Design review of the part built by this model. Coordinates are the model's own, in mm. Face numbers are marked on the shaded views. A direction names the side the tool comes from. Give positions to 0.01 mm unless a question says otherwise; leave off trailing zeros. Write each loop counter-clockwise with the first axis right and the second up, starting at its lowest first coordinate (ties: lowest second). Pieces come first, ordered by that corner, then holes.
```python
from build123d import *
from OCP.BRepFilletAPI import BRepFilletAPI_MakeChamfer

# Parameters (mm, degrees)
SKETCH1_R               = 1.5
BOSS_EXTRUDE1_DEPTH     = 21.8
CUT_EXTRUDE1_START      = -1.8
SKETCH2_W               = 54.830632019
SKETCH2_H               = 32.18582254
CUT_EXTRUDE1_DEPTH      = 1.8
SKETCH3_W               = 57.724078453
SKETCH3_H               = 32.716020725
CUT_EXTRUDE2_DEPTH      = 16.5
FILLET1_R               = 3
FILLET2_R               = 1
CUT_EXTRUDE3_DEPTH      = 17.8
CHAMFER1_SIZE           = 0.3
CHAMFER2_SIZE           = 1.5
SKETCH5_W               = 33.078515986
SKETCH5_H               = 22.592086676
CUT_EXTRUDE4_DEPTH      = 3
SKETCH6_W               = 2
SKETCH6_H               = 4
BOSS_EXTRUDE2_DEPTH     = 27
CHAMFER3_SIZE           = 3
CHAMFER3_SIZE2          = 1.273424449
CUT_EXTRUDE5_DEPTH      = 36.549578057
CUT_EXTRUDE5_DEPTH_BACK = 36.549578057
FILLET3_R               = 2


with BuildPart() as part:
    # Sketch1 → Boss-Extrude1 (new body)
    with BuildSketch(Plane.XY):
        with BuildLine():
            Line((1.791039749, 3.715784471), (10.476580913, 10.632270415))
            ThreePointArc((10.476580913, 10.632270415), (10.769573262, 10.79399958), (11.099519913, 10.85))
            Line((11.099519913, 10.85), (38.700480087, 10.85))
            ThreePointArc((38.700480087, 10.85), (39.030426738, 10.79399958), (39.323419087, 10.632270415))
            Line((39.323419087, 10.632270415), (48.008960251, 3.715784471))
            ThreePointArc((48.008960251, 3.715784471), (49.8, 0), (48.008960251, -3.715784471))
            Line((48.008960251, -3.715784471), (39.323419087, -10.632270415))
            ThreePointArc((39.323419087, -10.632270415), (39.030426738, -10.79399958), (38.700480087, -10.85))
            Line((38.700480087, -10.85), (11.099519913, -10.85))
            ThreePointArc((11.099519913, -10.85), (10.769573262, -10.79399958), (10.476580913, -10.632270415))
            Line((10.476580913, -10.632270415), (1.791039749, -3.715784471))
            ThreePointArc((1.791039749, -3.715784471), (0, 0), (1.791039749, 3.715784471))
        make_face()
        with Locations((4.9, 0)):
            Circle(SKETCH1_R, mode=Mode.SUBTRACT)
        with Locations((44.9, 0)):
            Circle(SKETCH1_R, mode=Mode.SUBTRACT)
    extrude(amount=BOSS_EXTRUDE1_DEPTH)

    # Sketch2 → Cut-Extrude1 (cut)
    with BuildSketch(Plane.XY.offset(21.8).offset(CUT_EXTRUDE1_START)):
        with Locations((23.298408534, -3.305326345)):
            Rectangle(SKETCH2_W, SKETCH2_H)
        with BuildLine():
            Line((11.099519913, -10.85), (38.700480087, -10.85))
            ThreePointArc((38.700480087, -10.85), (39.030426738, -10.79399958), (39.323419087, -10.632270415))
            Line((39.323419087, -10.632270415), (40.1, -10.013862089))
            Line((40.1, -10.013862089), (40.1, 10.013862089))
            Line((40.1, 10.013862089), (39.323419087, 10.632270415))
            ThreePointArc((39.323419087, 10.632270415), (39.030426738, 10.79399958), (38.700480087, 10.85))
            Line((38.700480087, 10.85), (11.099519913, 10.85))
            ThreePointArc((11.099519913, 10.85), (10.769573262, 10.79399958), (10.476580913, 10.632270415))
            Line((10.476580913, 10.632270415), (9.7, 10.013862089))
            Line((9.7, 10.013862089), (9.7, -10.013862089))
            Line((9.7, -10.013862089), (10.476580913, -10.632270415))
            ThreePointArc((10.476580913, -10.632270415), (10.769573262, -10.79399958), (11.099519913, -10.85))
        make_face(mode=Mode.SUBTRACT)
    extrude(amount=CUT_EXTRUDE1_DEPTH, mode=Mode.SUBTRACT)

    # Sketch3 → Cut-Extrude2 (cut)
    with BuildSketch(Plane(origin=(0, 0, 0), x_dir=(-1, 0, 0), z_dir=(0, 0, -1))):
        with Locations((-24.814355967, -1.741428677)):
            Rectangle(SKETCH3_W, SKETCH3_H)
        Polygon((-38.15, -9.05), (-38.15, 4.45), (-33.3, 9.25), (-16.5, 9.25), (-11.65, 4.45), (-11.65, -9.05), align=None, mode=Mode.SUBTRACT)
    extrude(amount=-CUT_EXTRUDE2_DEPTH, mode=Mode.SUBTRACT)

    # Fillet1
    fillet1_edges = [part.edges().sort_by_distance(p)[0] for p in [
        (38.15, -9.05, 8.25),
        (11.65, -9.05, 8.25),
    ]]
    fillet(fillet1_edges, radius=FILLET1_R)

    # Fillet2
    fillet2_edges = [part.edges().sort_by_distance(p)[0] for p in [
        (38.15, 4.45, 8.25),
        (33.3, 9.25, 8.25),
        (16.5, 9.25, 8.25),
        (11.65, 4.45, 8.25),
    ]]
    fillet(fillet2_edges, radius=FILLET2_R)

    # Sketch4 → Cut-Extrude3 (cut)
    with BuildSketch(Plane.XY.offset(21.8)):
        with BuildLine():
            Line((37.15, 4.032748035), (32.888818327, 8.25))
            Line((32.888818327, 8.25), (16.911181673, 8.25))
            Line((16.911181673, 8.25), (12.65, 4.032748035))
            Line((12.65, 4.032748035), (12.65, -6.05))
            ThreePointArc((12.65, -6.05), (13.235786438, -7.464213562), (14.65, -8.05))
            Line((14.65, -8.05), (35.15, -8.05))
            ThreePointArc((35.15, -8.05), (36.564213562, -7.464213562), (37.15, -6.05))
            Line((37.15, -6.05), (37.15, 4.032748035))
        make_face()
    extrude(amount=-CUT_EXTRUDE3_DEPTH, mode=Mode.SUBTRACT)

    # Chamfer1
    chamfer1_edges = [part.edges().sort_by_distance(p)[0] for p in [
        (37.15, -1.008625983, 21.8),
        (35.019409163, 6.141374017, 21.8),
        (24.9, 8.25, 21.8),
        (14.780590837, 6.141374017, 21.8),
        (12.65, -1.008625983, 21.8),
        (13.235786438, -7.464213562, 21.8),
        (24.9, -8.05, 21.8),
        (36.564213562, -7.464213562, 21.8),
    ]]
    chamfer(chamfer1_edges, length=CHAMFER1_SIZE)

    # Chamfer2
    chamfer2_edges = [part.edges().sort_by_distance(p)[0] for p in [
        (3.4, 0, 20),
        (43.4, 0, 20),
    ]]
    chamfer(chamfer2_edges, length=CHAMFER2_SIZE)

    # Sketch5 → Cut-Extrude4 (cut)
    with BuildSketch(Plane(origin=(0, 0, 0), x_dir=(-1, 0, 0), z_dir=(0, 0, -1))):
        with Locations((-24.236330555, -0.057007702)):
            Rectangle(SKETCH5_W, SKETCH5_H)
        with BuildLine():
            Line((-26.875, -1.55), (-22.925, -1.55))
            ThreePointArc((-22.925, -1.55), (-22.571446609, -1.403553391), (-22.425, -1.05))
            Line((-22.425, -1.05), (-22.425, 7.95))
            ThreePointArc((-22.425, 7.95), (-22.571446609, 8.303553391), (-22.925, 8.45))
            Line((-22.925, 8.45), (-26.875, 8.45))
            ThreePointArc((-26.875, 8.45), (-27.228553391, 8.303553391), (-27.375, 7.95))
            Line((-27.375, 7.95), (-27.375, -1.05))
            ThreePointArc((-27.375, -1.05), (-27.228553391, -1.403553391), (-26.875, -1.55))
        make_face(mode=Mode.SUBTRACT)
        with BuildLine():
            Line((-19.9, -8.25), (-15.95, -8.25))
            ThreePointArc((-15.95, -8.25), (-15.596446609, -8.103553391), (-15.45, -7.75))
            Line((-15.45, -7.75), (-15.45, 1.25))
            ThreePointArc((-15.45, 1.25), (-15.596446609, 1.603553391), (-15.95, 1.75))
            Line((-15.95, 1.75), (-19.9, 1.75))
            ThreePointArc((-19.9, 1.75), (-20.253553391, 1.603553391), (-20.4, 1.25))
            Line((-20.4, 1.25), (-20.4, -7.75))
            ThreePointArc((-20.4, -7.75), (-20.253553391, -8.103553391), (-19.9, -8.25))
        make_face(mode=Mode.SUBTRACT)
        with BuildLine():
            Line((-33.85, -8.25), (-29.9, -8.25))
            ThreePointArc((-29.9, -8.25), (-29.546446609, -8.103553391), (-29.4, -7.75))
            Line((-29.4, -7.75), (-29.4, 1.25))
            ThreePointArc((-29.4, 1.25), (-29.546446609, 1.603553391), (-29.9, 1.75))
            Line((-29.9, 1.75), (-33.85, 1.75))
            ThreePointArc((-33.85, 1.75), (-34.203553391, 1.603553391), (-34.35, 1.25))
            Line((-34.35, 1.25), (-34.35, -7.75))
            ThreePointArc((-34.35, -7.75), (-34.203553391, -8.103553391), (-33.85, -8.25))
        make_face(mode=Mode.SUBTRACT)
    extrude(amount=-CUT_EXTRUDE4_DEPTH, mode=Mode.SUBTRACT)

    # Sketch6 → Boss-Extrude2 (add)
    with BuildSketch(Plane.XY.offset(20)):
        with Locations((24.9, 3.45)):
            Rectangle(SKETCH6_W, SKETCH6_H)
        with Locations((17.925, -3.25)):
            Rectangle(SKETCH6_W, SKETCH6_H)
        with Locations((31.875, -3.25)):
            Rectangle(SKETCH6_W, SKETCH6_H)
    extrude(amount=-BOSS_EXTRUDE2_DEPTH)

    # Chamfer3: one chamfer whose edges measure the first distance from different faces: ONE call of the kernel's chamfer builder (chamfer() names one face for all edges)
    chamfer3_edges_1 = [part.edges().sort_by_distance(p)[0] for p in [
        (24.9, 1.45, 20),
    ]]
    chamfer3_side_1 = [part.faces().sort_by_distance(p)[0] for p in [
        (24.9, 1.45, 12),
    ]]
    chamfer3_edges_2 = [part.edges().sort_by_distance(p)[0] for p in [
        (24.9, 5.45, 20),
    ]]
    chamfer3_side_2 = [part.faces().sort_by_distance(p)[0] for p in [
        (24.9, 5.45, 12),
    ]]
    chamfer3_edges_3 = [part.edges().sort_by_distance(p)[0] for p in [
        (17.925, -5.25, 20),
    ]]
    chamfer3_side_3 = [part.faces().sort_by_distance(p)[0] for p in [
        (17.925, -5.25, 12),
    ]]
    chamfer3_edges_4 = [part.edges().sort_by_distance(p)[0] for p in [
        (17.925, -1.25, 20),
    ]]
    chamfer3_side_4 = [part.faces().sort_by_distance(p)[0] for p in [
        (17.925, -1.25, 12),
    ]]
    chamfer3_edges_5 = [part.edges().sort_by_distance(p)[0] for p in [
        (31.875, -5.25, 20),
    ]]
    chamfer3_side_5 = [part.faces().sort_by_distance(p)[0] for p in [
        (31.875, -5.25, 12),
    ]]
    chamfer3_edges_6 = [part.edges().sort_by_distance(p)[0] for p in [
        (31.875, -1.25, 20),
    ]]
    chamfer3_side_6 = [part.faces().sort_by_distance(p)[0] for p in [
        (31.875, -1.25, 12),
    ]]
    chamfer3 = BRepFilletAPI_MakeChamfer(part.part.solid().wrapped)
    for e in chamfer3_edges_1:
        chamfer3.Add(CHAMFER3_SIZE, CHAMFER3_SIZE2, e.wrapped, chamfer3_side_1[0].wrapped)  # the first distance lies on this face
    for e in chamfer3_edges_2:
        chamfer3.Add(CHAMFER3_SIZE, CHAMFER3_SIZE2, e.wrapped, chamfer3_side_2[0].wrapped)  # the first distance lies on this face
    for e in chamfer3_edges_3:
        chamfer3.Add(CHAMFER3_SIZE, CHAMFER3_SIZE2, e.wrapped, chamfer3_side_3[0].wrapped)  # the first distance lies on this face
    for e in chamfer3_edges_4:
        chamfer3.Add(CHAMFER3_SIZE, CHAMFER3_SIZE2, e.wrapped, chamfer3_side_4[0].wrapped)  # the first distance lies on this face
    for e in chamfer3_edges_5:
        chamfer3.Add(CHAMFER3_SIZE, CHAMFER3_SIZE2, e.wrapped, chamfer3_side_5[0].wrapped)  # the first distance lies on this face
    for e in chamfer3_edges_6:
        chamfer3.Add(CHAMFER3_SIZE, CHAMFER3_SIZE2, e.wrapped, chamfer3_side_6[0].wrapped)  # the first distance lies on this face
    add(Compound.cast(chamfer3.Shape()), mode=Mode.REPLACE)

    # Sketch7 → Cut-Extrude5 (cut, two sides: drawn at the far end of the back side and taken through both)
    with BuildSketch(Plane(origin=(25.9, 0, 0), x_dir=(0, 0, -1), z_dir=(1, 0, 0)).offset(-CUT_EXTRUDE5_DEPTH_BACK)):
        with BuildLine():
            Line((3.15, 4.3), (5.15, 4.3))
            ThreePointArc((5.15, 4.3), (6, 3.45), (5.15, 2.6))
            Line((5.15, 2.6), (3.15, 2.6))
            ThreePointArc((3.15, 2.6), (2.3, 3.45), (3.15, 4.3))
        make_face()
        with BuildLine():
            Line((3.15, -2.4), (5.15, -2.4))
            ThreePointArc((5.15, -2.4), (6, -3.25), (5.15, -4.1))
            Line((5.15, -4.1), (3.15, -4.1))
            ThreePointArc((3.15, -4.1), (2.3, -3.25), (3.15, -2.4))
        make_face()
    extrude(amount=CUT_EXTRUDE5_DEPTH + CUT_EXTRUDE5_DEPTH_BACK, mode=Mode.SUBTRACT)

    # Fillet3
    fillet3_edges = [part.edges().sort_by_distance(p)[0] for p in [
        (31.875, -5.25, -7),
        (31.875, -1.25, -7),
        (17.925, -5.25, -7),
        (24.9, 1.45, -7),
        (17.925, -1.25, -7),
        (24.9, 5.45, -7),
    ]]
    fillet(fillet3_edges, radius=FILLET3_R - 0.0001)  # a hair under: the kernel refuses the full size


solid = part.part
```
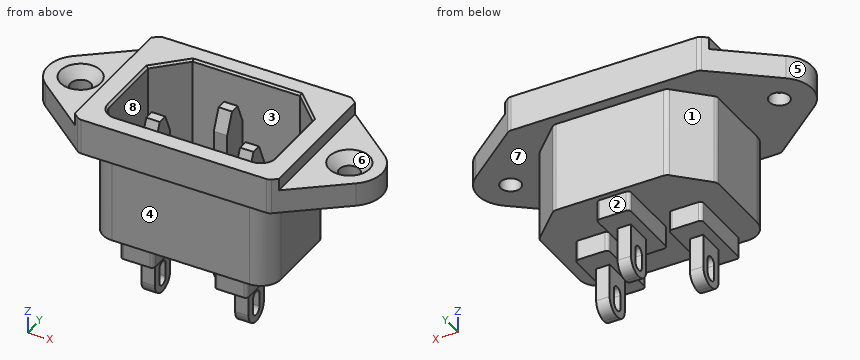
(1) To check wall thickness, follow L1, parallel to Y at x = 24, z = 6; L2, parallel to Y at x = 27.5, z = 20.25; L3, parallel to Y at x = 30.5, z = 11.75. State the ranges of each line that lie inside material, in increasing order.
Resolved:
L1: y = -9.05 to -8.05, 1.45 to 5.45, 8.25 to 9.25
L2: y = -10.85 to -8.05, 8.25 to 10.85
L3: y = -9.05 to -8.05, 8.25 to 9.25
(2) Mouldability with a two-part tool opening along Y and no side actions: class the marked faces 5, 6, 7 and 8 as pulls with the +Y half, pulls with the -Y half, needs draft (parallel to the pull), parting line crosses it, or undercut.
Resolved:
face 5: parting line crosses it
face 6: undercut
face 7: needs draft
face 8: undercut
(3) Consider section B-B, the plane z = 13.75. Give the number of separate pieces and of enclosed holes in the cut face, then the cut area to 3 significant figures.
Resolved:
separate pieces: 4
enclosed holes: 1
area: 102 mm2
(4) Clearance check with flat-ended pins moving along their axes: P1, Ø0.6, axis at x = 25, z = -2.5, coming from the -Y side; P2, Ø3.5, axis at x = 44.9, y = 0, coming from the +Z side; P3, Ø3, axis at y = -1, z = 10, coming from the -X side. State where each tip first meets the part, or that it passes through.
Resolved:
P1: stops at y = 1.45
P2: stops at z = 18.75
P3: stops at x = 11.65
(5) Consider section A-A, the plane z = -1.75. Give the boundary of the cut face in (x, y) (3 decimals).
Resolved:
outline: (16.925, -5.25) - (18.925, -5.25) - (18.925, -1.25) - (16.925, -1.25) - close; (23.9, 1.45) - (25.9, 1.45) - (25.9, 5.45) - (23.9, 5.45) - close; (30.875, -5.25) - (32.875, -5.25) - (32.875, -1.25) - (30.875, -1.25) - close
(6) Tool access review of the marked faces 1, 2, 3 and 4: name each direction out of +Z, -Z, +X, -X, +Y, -Y from which nothing blocks a thin tool from reaching the whole face with its end or side.
Resolved:
face 1: -Z, -X, +Y
face 2: -Z, +X, -X, +Y
face 3: +Z
face 4: -Z, +X, -X, -Y
(7) Consider section C-C, the plane x = 44.9. Give the boundary of the cut face in (y, z), then the cut area to 3 significant figures.
Resolved:
outline: (-6.19, 16.5) - (-1.5, 16.5) - (-1.5, 18.5) - (-3, 20) - (-6.19, 20) - close; (1.5, 16.5) - (6.19, 16.5) - (6.19, 20) - (3, 20) - (1.5, 18.5) - close
area: 30.6 mm2
